```python
from build123d import *

# Parameters (mm, degrees)
F0_W      = 54
F0_H      = 34
F1_DEPTH  = 14
F2_W      = 14
F2_H      = 34
F3_DEPTH  = 14
F5_DEPTH  = 14
F7_DEPTH  = 14
F8_R      = 7
F9_DEPTH  = 25
F11_DEPTH = 25


with BuildPart() as f1:
    # F0 (on Top) → F1 (new body)
    with BuildSketch(Plane.XY):
        with Locations((-1.2663472444, 3.4664713239)):
            Rectangle(F0_W, F0_H)
    extrude(amount=F1_DEPTH)

    # F2 (on face) → F3 (join)
    with BuildSketch(Plane.XY.offset(14)):
        with Locations((18.7336527556, 3.4664713239)):
            Rectangle(F2_W, F2_H)
    extrude(amount=F3_DEPTH)

    # F4 (on face) → F5 (join)
    with BuildSketch(Plane.YZ.offset(25.7336527556)):
        with BuildLine():
            Line((-13.5335286761, 28), (20.4664713239, 28))
            ThreePointArc((20.4664713239, 28), (3.4664713239, 45), (-13.5335286761, 28))
        make_face()
        with BuildLine():
            ThreePointArc((-13.5335286761, 28), (3.4664713239, 11), (20.4664713239, 28))
            Line((20.4664713239, 28), (-13.5335286761, 28))
        make_face()
    extrude(amount=-F5_DEPTH)

    # F6 (on face) → F7 (join)
    with BuildSketch(Plane.XY.offset(14)):
        with BuildLine():
            Line((-28.2663472444, -13.5335286761), (-28.2663472444, 20.4664713239))
            ThreePointArc((-28.2663472444, 20.4664713239), (-45.2663472444, 3.4664713239), (-28.2663472444, -13.5335286761))
        make_face()
    extrude(amount=-F7_DEPTH)

    # F8 (on face) → F9 (cut)
    with BuildSketch(Plane.YZ.offset(25.7336527556)):
        with Locations((3.4664713239, 28)):
            Circle(F8_R)
    extrude(amount=-F9_DEPTH, mode=Mode.SUBTRACT)

    # F10 (on face) → F11 (cut)
    with BuildSketch(Plane.XY.offset(14)):
        with BuildLine():
            ThreePointArc((-27.9110185812, -3.5245043978), (-23.1925271529, -1.3560124427), (-21.2663472444, 3.4664713239))
            ThreePointArc((-21.2663472444, 3.4664713239), (-23.3165997761, 8.4162187922), (-28.2663472444, 10.4664713239))
            ThreePointArc((-28.2663472444, 10.4664713239), (-35.2640908111, 3.2887497041), (-27.9110185812, -3.5245043978))
        make_face()
        with BuildLine():
            ThreePointArc((-28.2663472444, 10.4664713239), (-23.3165997761, 8.4162187922), (-21.2663472444, 3.4664713239))
            ThreePointArc((-21.2663472444, 3.4664713239), (-23.1925271529, -1.3560124427), (-27.9110185812, -3.5245043978))
            Line((-27.9110185812, -3.5245043978), (-4.2690190308, -3.5335281663))
            ThreePointArc((-4.2690190308, -3.5335281663), (-11.2663471169, 3.4678072171), (-4.2663472444, 10.4664713239))
            Line((-4.2663472444, 10.4664713239), (-28.2663472444, 10.4664713239))
        make_face()
        with BuildLine():
            ThreePointArc((2.7336527556, 3.4664713239), (0.6834002239, 8.4162187922), (-4.2663472444, 10.4664713239))
            ThreePointArc((-4.2663472444, 10.4664713239), (-11.2663471169, 3.4678072171), (-4.2690190308, -3.5335281663))
            ThreePointArc((-4.2690190308, -3.5335281663), (0.6824555146, -1.4842206735), (2.7336527556, 3.4664713239))
        make_face()
    extrude(amount=-F11_DEPTH, mode=Mode.SUBTRACT)


solid = f1.part
```
Can you work these out from the model? Positions are in its coordinate system, mm. A direction names the side the tool comes from. Give positions to 0.01 mm unless a question says otherwise; leave off trailing zeros. Loops run counter-clockwise (first coordinate to the right, second up) from the corner with the lowest first, then second, coordinate; pieces in that order, holes last. Notation, with made-up numbers: M 54,51 L 83,51 A13 ccw 83,60 Z; hole C 0.5,87.25 d4. An arc over 180 degrees is marked long. One line per item, written item: value.
(1) Suppose I cut it at B-B on x = 19. List the corners of the cut face in (y, z) for me.
Returned:
outline: M -13.53,0 L 20.47,0 L 20.47,28 A17 ccw -13.53,28 Z; hole C 3.47,28 d14
(2) Will these pins go through, and if not, where does the flat tip stop? pin 1 (6 mm diameter, centred on x = 7.5, z = 23, fed in from +Y); pin 2 (18 mm diameter, centred on y = 3.47, z = 28, fed in from -X); pin 3 (10 mm diameter, centred on x = -10.5, y = 14.5, fed in from +Z); pin 4 (6 mm diameter, centred on x = 16, y = 15.5, fed in from +Z).
Returned:
pin 1: through
pin 2: x = 11.73
pin 3: z = 14
pin 4: z = 42.4
(3) We'd pull the mould along Y, two halves only. Please class faces 1 (the face through (25.734, 3, 18)), 2 (the face through (-45.262, 3.84, 7.098)), 3 (the face through (-35.266, 3.445, 7.098)): released by +Y, released by -Y, zero draft, split by the parting line, or undercut.
Returned:
face 1: zero draft
face 2: split by the parting line
face 3: undercut
(4) Suppose I cut it at C-C on x = -3.5. List the corners of the cut face in (y, z) for me.
Returned:
outline: M -13.53,0 L -3.49,0 L -3.49,14 L -13.53,14 Z; M 10.42,0 L 20.47,0 L 20.47,14 L 10.42,14 Z
(5) Which directions (+Z, -Z, +X, -X, +Y, -Y) give clear straight access to the entire face, cutting with the end or side of a thin tool? Please do faces 4 (the face through (11.734, -4, 30)), 5 (the face through (18.832, 1.949, 21.166)), 6 (the face through (-16, 10.466, 7)).
Returned:
face 4: +Z, -X, +Y, -Y
face 5: +X, -X
face 6: +Z, -Z
(6) Suppose I cut it at D-D on z = 29. List the corners of the cut face in (x, y) for me.
Returned:
outline: M 11.73,-13.5 L 25.73,-13.5 L 25.73,-3.46 L 11.73,-3.46 Z; M 11.73,10.39 L 25.73,10.39 L 25.73,20.44 L 11.73,20.44 Z
(7) I need wall thicknesses on line 1 (Z direction, x = -0.5, y = 15.5); line 2 (X direction, y = 3, z = 7); line 3 (X direction, y = -2, z = 42). Which ranges of each line are inside material? Lowest first, please.
Returned:
line 1: 0 to 14
line 2: -45.26 to -35.25, 2.72 to 25.73
line 3: 11.73 to 25.73
(8) Suppose I cut it at A-A on z = 10.5. List the corners of the cut face in (x, y) for me, plus the area to 3 significant figures.
Returned:
outline: M -28.27,-13.53 L 25.73,-13.53 L 25.73,20.47 L -28.27,20.47 A17 ccw Z; hole M -28.27,10.47 A7 ccw long -27.91,-3.52 L -4.27,-3.53 A7 ccw -4.27,10.47 Z
area: 1,800 mm^2
